Read the model definition and answer for the solid it produces. Units are mm, in the model's axes. Give positions to 0.01 mm unless a question says otherwise; leave off trailing zeros. Order: outer loops, then holes, each group sorted by start corner. A loop starts at its lowest first (then second) coordinate and runs counter-clockwise, first axis right, second up.
```python
from build123d import *

# Parameters (mm, degrees)
SKETCH_1_W          = 85
SKETCH_1_H          = 85
EXTRUDE_1_DEPTH     = 70
SKETCH_2_R          = 25
CUT_EXTRUDE_1_DEPTH = 140


with BuildPart() as part:
    # 草图1 → 凸台-拉伸1 (new, symmetric)
    with BuildSketch(Plane(origin=(0, 0, 0), x_dir=(1, 0, 0), z_dir=(0, 1, 0))):
        Rectangle(SKETCH_1_W, SKETCH_1_H)
    extrude(amount=EXTRUDE_1_DEPTH, both=True)

    # 草图2 → 切除-拉伸1 (cut)
    with BuildSketch(Plane(origin=(0, 70, 0), x_dir=(1, 0, 0), z_dir=(0, 1, 0))):
        with Locations(Location((0, 0, 0), (0, 0, 270))):
            Circle(SKETCH_2_R)
    extrude(amount=-CUT_EXTRUDE_1_DEPTH, mode=Mode.SUBTRACT)


solid = part.part
```
1) The part is cut by section C-C on y = -28.5. Determine the outline of the cut face in (x, z).
Final values:
outline: (-42.5, -42.5) - (42.5, -42.5) - (42.5, 42.5) - (-42.5, 42.5) - close; hole circle Ø50 at (0, 0)
2) The part is cut by section B-B on z = 0. Determine the outline of the cut face in (x, y), and give its area (3 significant figures).
Final values:
outline: (-42.5, -70) - (-25, -70) - (-25, 70) - (-42.5, 70) - close; (25, -70) - (42.5, -70) - (42.5, 70) - (25, 70) - close
area: 4,900 mm2
3) The part is cut by section A-A on x = -20. Determine the outline of the cut face in (y, z).
Final values:
outline: (-70, -42.5) - (70, -42.5) - (70, -15) - (-70, -15) - close; (-70, 15) - (70, 15) - (70, 42.5) - (-70, 42.5) - close
4) Consider L1, parallel to X at y = 16, z = 0.5 (3 decimals); L2, parallel to X at y = 23, z = 19; L3, parallel to Z at x = -14.5, y = 5. Determine where each line is inside the solid, lowest interval first.
Final values:
L1: x = -42.5 to -24.995, 24.995 to 42.5
L2: x = -42.5 to -16.25, 16.25 to 42.5
L3: z = -42.5 to -20.37, 20.37 to 42.5
5) For a pull along X with two mould halves and no side action, classify faces 1 (the face through (-1, 1, 42.5)), 2 (the face through (7.509, 0.98, 23.846)), 3 (the face through (-42.5, 1, 1)), 4 (the face through (42.5, 1, 1)) as released by +X, released by -X, zero draft, split by the parting line, or undercut.
Final values:
face 1: zero draft
face 2: undercut
face 3: released by -X
face 4: released by +X
